from build123d import *

# Parameters (mm, degrees)
SKETCH_1_R      = 6.725
SKETCH_1_R_2    = 4.68
EXTRUDE_1_DEPTH = 2.4
SKETCH_2_R      = 2
EXTRUDE_2_DEPTH = 107.5
SKETCH_4_R      = 3
EXTRUDE_3_DEPTH = 100


with BuildPart() as part:
    # 스케치1 → 보스-돌출1 (new body, symmetric)
    with BuildSketch(Plane(origin=(0, 0, 0), x_dir=(1, 0, 0), z_dir=(0, 1, 0))):
        Circle(SKETCH_1_R)
        Circle(SKETCH_1_R_2, mode=Mode.SUBTRACT)
    extrude_1 = extrude(amount=EXTRUDE_1_DEPTH, both=True)

    # 스케치2 → 보스-돌출2 (add, symmetric)
    with BuildSketch(Plane.XY.offset(113.45)):
        Circle(SKETCH_2_R)
    extrude(amount=EXTRUDE_2_DEPTH, both=True)

    # 대칭 복사5: 보스-돌출1 across plane
    add(extrude_1.mirror(Plane.XY.offset(113.45)))

    # 스케치4 → 보스-돌출3 (add, symmetric)
    with BuildSketch(Plane.XY.offset(113.45)):
        Circle(SKETCH_4_R)
    extrude(amount=EXTRUDE_3_DEPTH, both=True)


solid = part.part
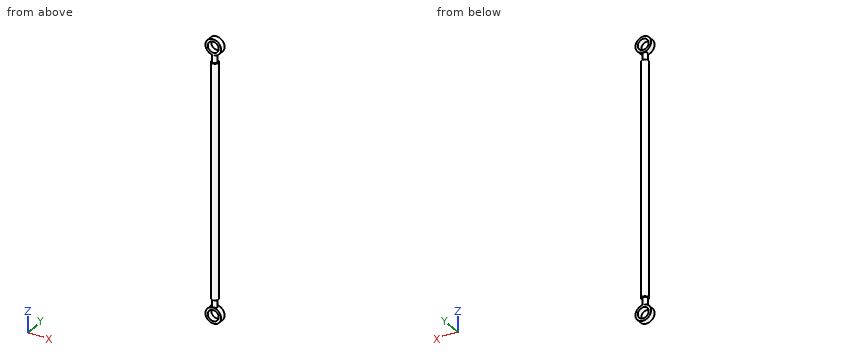
Design review of the part built by this model. Coordinates are the model's own, in mm. Coordinates: 2 decimals unless noted, no trailing zeros. Write each loop counter-clockwise with the first axis right and the second up, starting at its lowest first coordinate (ties: lowest second). Pieces come first, ordered by that corner, then holes. Notation, with made-up numbers: (74, 58.25) - (81, 58.25) arc R20 cw to (81, 84.25) - close; hole circle Ø6 at (48, -22.75). An arc over 180 degrees is marked (long way). Use one line per item in the form item = value.
Q1. Consider section C-C (z = 226.9). Write out the cut boundary in (x, y) (3 decimals), plus the area to 3 significant figures.
Taken from the geometry:
outline = (-6.725, -2.4) - (-4.68, -2.4) - (-4.68, 2.4) - (-6.725, 2.4) - close; (4.68, -2.4) - (6.725, -2.4) - (6.725, 2.4) - (4.68, 2.4) - close
area = 19.6 mm^2
Q2. Consider section D-D (z = 78). Write out the cut boundary in (x, y).
Taken from the geometry:
outline = circle Ø6 at (0, 0)
Q3. Insertion check: pin 1 Ø4 at (x, z) = (1, 226) entering from -Y; pin 2 Ø1.8 at (x, y) = (0.5, -1) entering from +Z (3 decimals); pin 3 Ø3 at (x, z) = (2, 113) entering from +Y; pin 4 Ø1 at (x, y) = (-2.5, 0) entering from -Z. Each pin has a flat end and moves straight along its axis. Give the tip position at first contact, or say it passes through.
Taken from the geometry:
pin_1 = through
pin_2 = 233.625
pin_3 = 2.96
pin_4 = -6.42
Q4. Consider section A-A (x = 0). Write out the cut boundary in (y, z) (3 decimals), plus the area to 3 significant figures.
Taken from the geometry:
outline = (-3, 13.45) - (-2, 13.45) - (-2, 6.725) - (-2.4, 6.725) - (-2.4, 4.68) - (2.4, 4.68) - (2.4, 6.725) - (2, 6.725) - (2, 13.45) - (3, 13.45) - (3, 213.45) - (2, 213.45) - (2, 220.175) - (2.4, 220.175) - (2.4, 222.22) - (-2.4, 222.22) - (-2.4, 220.175) - (-2, 220.175) - (-2, 213.45) - (-3, 213.45) - close; (-2.4, -6.725) - (2.4, -6.725) - (2.4, -4.68) - (-2.4, -4.68) - close; (-2.4, 231.58) - (2.4, 231.58) - (2.4, 233.625) - (-2.4, 233.625) - close
area = 1,290 mm^2
Q5. Consider section B-B (y = 0). Write out the cut boundary in (x, z) (3 decimals), plus the area to 3 significant figures.
Taken from the geometry:
outline = (-3, 13.45) - (-2, 13.45) - (-2, 6.421) arc R6.725 ccw (long way) to (2, 6.421) - (2, 13.45) - (3, 13.45) - (3, 213.45) - (2, 213.45) - (2, 220.479) arc R6.725 ccw (long way) to (-2, 220.479) - (-2, 213.45) - (-3, 213.45) - close; hole circle Ø9.36 at (0, 0); hole circle Ø9.36 at (0, 226.9)
area = 1,400 mm^2
Q6. For probe 1 along Z at (x, y) = (0, -0.05) (3 decimals); probe 2 along Z at (x, y) = (0, 2.15) (3 decimals); probe 3 along Z at (x, y) = (-0.75, 0.1), list the stretches that pass through material, from the lowest coordinate up.
Taken from the geometry:
probe_1 = -6.725 to -4.68, 4.68 to 222.22, 231.58 to 233.625
probe_2 = -6.725 to -4.68, 4.68 to 6.725, 13.45 to 213.45, 220.175 to 222.22, 231.58 to 233.625
probe_3 = -6.68 to -4.62, 4.62 to 222.28, 231.52 to 233.58
